Check sheet for the drawn part. Datum: minimum x, y, z corner. Units: mm. Coordinates: 2 decimals unless noted, no trailing zeros. Write each loop counter-clockwise with the first axis right and the second up, starting at its lowest first coordinate (ties: lowest second). Pieces come first, ordered by that corner, then holes. Notation, with made-up numbers: M 48,-11 L 69,-11 A7 ccw 69,-2 Z; hole C 12,12.5 d1. An arc over 180 degrees is marked long. Answer in a Markdown table with one row per item.
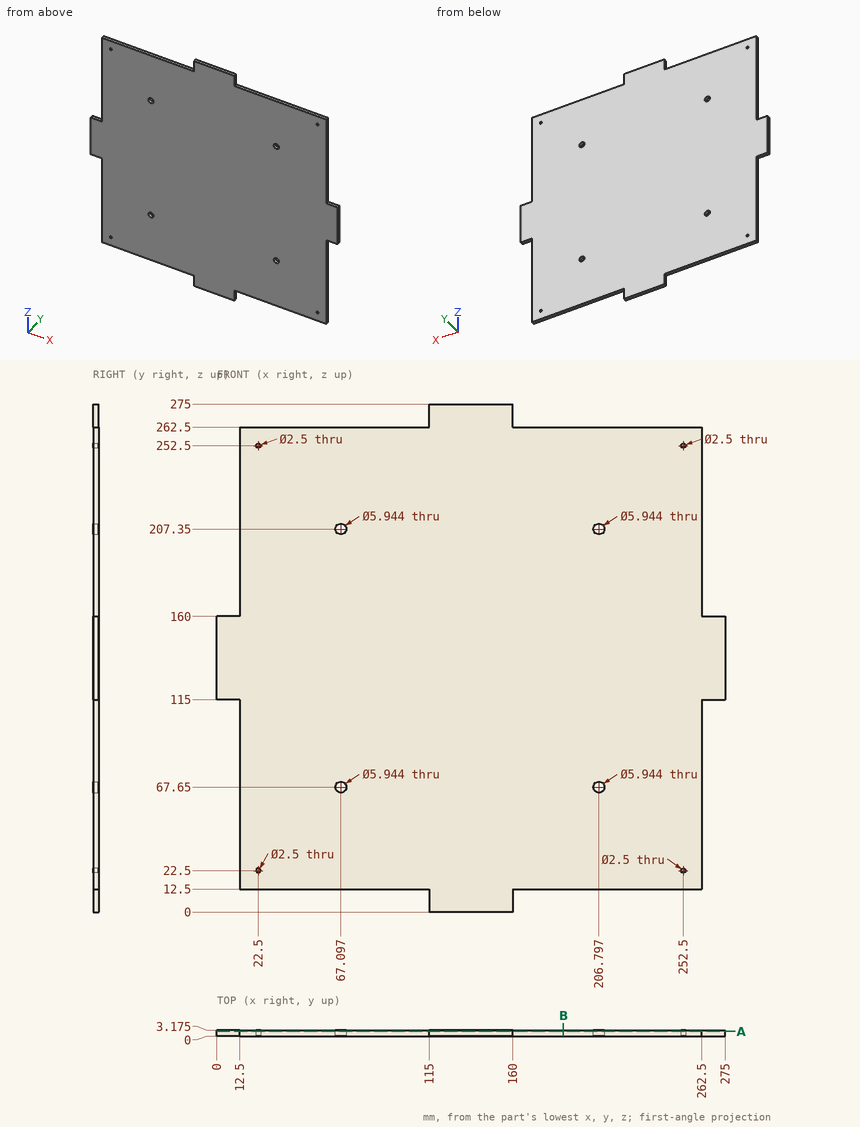
1) Thickness scan on L1, parallel to X at y = 1, z = 22.5; L2, parallel to X at y = 2.35, z = 67.65 (1 decimal); L3, parallel to Z at x = 14, y = 1.25. Record the ranges inside material, lowest first. Write a range as [from, to].
Response values:
| item | result |
|---|---|
| L1 | x = [12.5, 21.25], [23.75, 251.25], [253.75, 262.5] |
| L2 | x = [12.5, 64.1], [70.1, 203.8], [209.8, 262.5] |
| L3 | z = [12.5, 262.5] |
2) Sectioned sample at A-A (y = 2.5). Give the number of separate pieces and of enclosed holes in the cut face, then the cut area to 3 significant figures.
Response values:
| item | result |
|---|---|
| separate pieces | 1 |
| enclosed holes | 8 |
| area | 64,600 mm² |
3) Sectioned sample at B-B (x = 187.5). Record the cut outline in (y, z) (1 decimal).
Response values:
| item | result |
|---|---|
| outline | M 0,12.5 L 3.2,12.5 L 3.2,262.5 L 0,262.5 Z |
4) Depth check by flat-ended pin: pin 1 (1 mm diameter, centred on y = 2, z = 271, fed in from +X); pin 2 (2 mm diameter, centred on x = 252.5, z = 22.5, fed in from +Y); pin 3 (1.6 mm diameter, centred on y = 2, z = 67.5, fed in from +X); pin 4 (7 mm diameter, centred on x = 206.8, z = 207.35, fed in from +Y) (3 decimals). Enter the tip coordinate at first touch or a pass-through.
Response values:
| item | result |
|---|---|
| pin 1 | stops at x = 160 |
| pin 2 | passes through |
| pin 3 | stops at x = 262.5 |
| pin 4 | stops at y = 3.175 |
